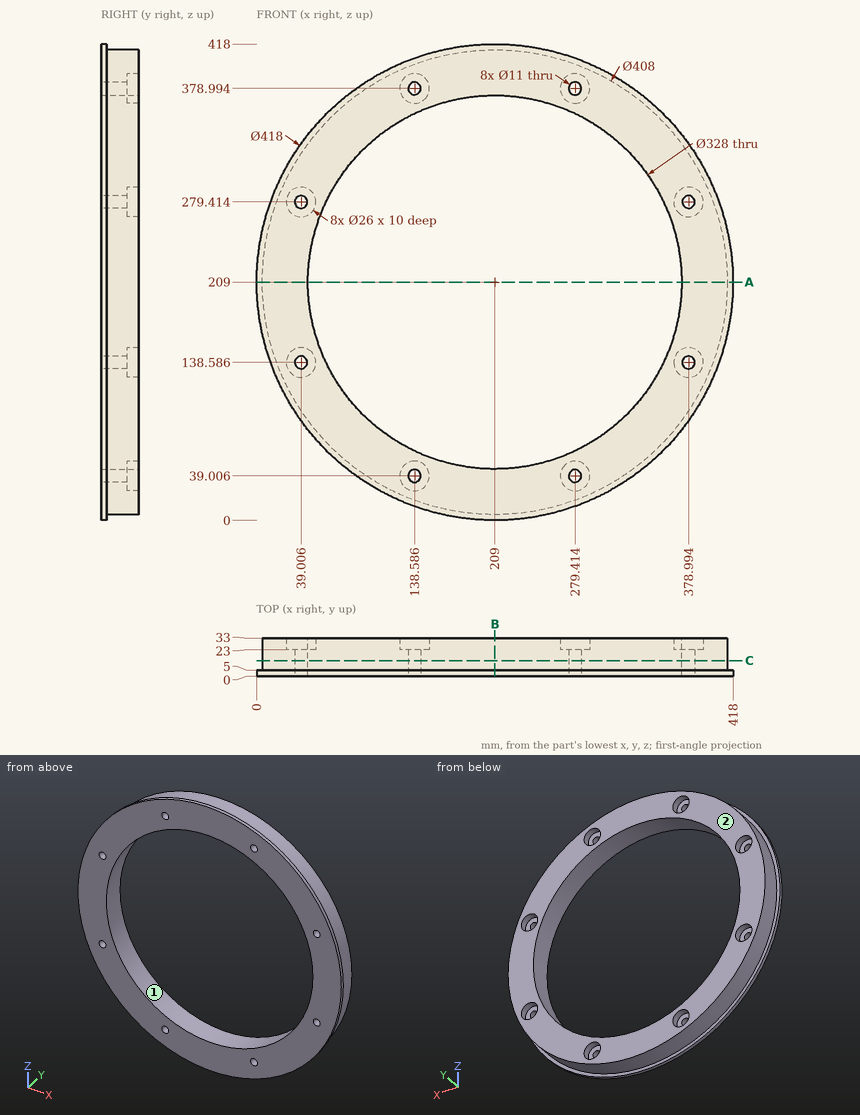
Design review of the part shown in the three views and the two pictorial views. Dimensions are in mm from the part's minimum x, y and z. Round coordinates to 2 decimals unless told otherwise and drop trailing zeros. Loops run counter-clockwise (first coordinate to the right, second up) from the corner with the lowest first, then second, coordinate; pieces in that order, holes last. Notation, with made-up numbers: (-20.5, 53) -> (-0.5, 53) arc R23 ccw to (-0.5, 66) -> close; hole circle Ø2 at (70, 3.25). An arc over 180 degrees is marked (long way). Return JSON: item names as keys, results as strings.
(1) For line 1 (Z direction, x = 268.5, y = 25.5) (1 decimal); line 2 (X direction, y = 15, z = 380) (1 decimal); line 3 (X direction, y = 29, z = 43) (1 decimal), list the stretches that pass through material, from the lowest coordinate up.
Solved:
{"line 1": "13.9 to 31.9, 46.1 to 56.2, 361.8 to 371.9, 386.1 to 404.1", "line 2": "97.8 to 133.2, 144 to 274, 284.8 to 320.2", "line 3": "90.4 to 126.2, 151 to 267, 291.8 to 327.6"}
(2) The part is to be moulded in two halves that separate along Z. For the marked faces 1 and 2, say which applies: released by +Z, released by -Z, zero draft, split by the parting line, or undercut.
Solved:
{"face 1": "undercut", "face 2": "zero draft"}
(3) For pin 1 (12.5 mm diameter, centred on x = 39.01, z = 279.41, fed in from +Y); pin 2 (10 mm diameter, centred on x = 279.41, z = 39.01, fed in from -Y) (3 decimals); pin 3 (6 mm diameter, centred on x = 311.5, y = 28.5, fed in from +Z); pin 4 (2 mm diameter, centred on y = 21.5, z = 54.5, fed in from -X) (1 decimal), all flat-tipped, find the tip position at first contact; note any pin that passes through.
Solved:
{"pin 1": "y = 23", "pin 2": "through", "pin 3": "z = 387.09", "pin 4": "x = 74.6"}
(4) Add section B-B on x = 209. Write out the cut boundary in (y, z), plus the area to 3 significant figures.
Solved:
{"outline": "(0, 0) -> (5, 0) -> (5, 5) -> (33, 5) -> (33, 45) -> (0, 45) -> close; (0, 373) -> (33, 373) -> (33, 413) -> (5, 413) -> (5, 418) -> (0, 418) -> close", "area": "2,690 mm2"}
(5) Add section C-C on y = 13.5. State how many separate pieces and enclosed holes the cut face has, plus the area to 3 significant figures.
Solved:
{"separate pieces": "1", "enclosed holes": "9", "area": "45,500 mm2"}
(6) Add section A-A on z = 209. Write out the cut boundary in (x, y), plus the area to 3 significant figures.
Solved:
{"outline": "(0, 0) -> (45, 0) -> (45, 33) -> (5, 33) -> (5, 5) -> (0, 5) -> close; (373, 0) -> (418, 0) -> (418, 5) -> (413, 5) -> (413, 33) -> (373, 33) -> close", "area": "2,690 mm2"}
